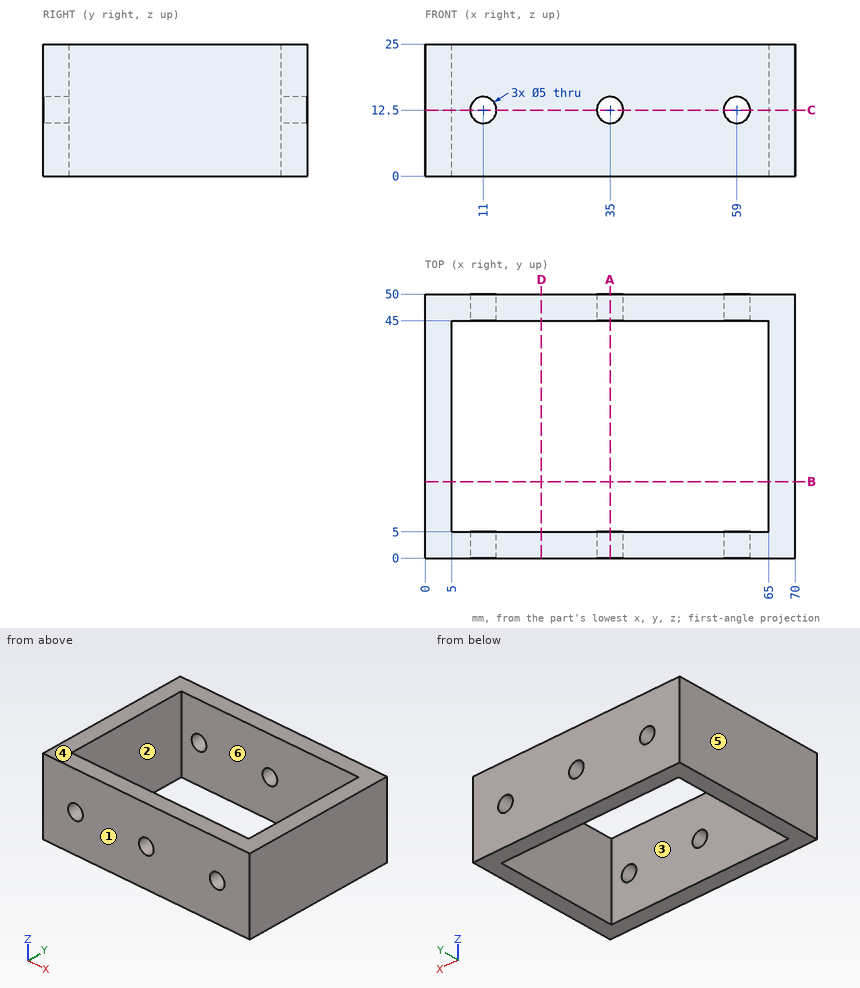
Design review of the part shown in the three views and the two pictorial views. Dimensions are in mm from the part's minimum x, y and z. A direction names the side the tool comes from. Give positions to 0.01 mm unless a question says otherwise; leave off trailing zeros. Loops run counter-clockwise (first coordinate to the right, second up) from the corner with the lowest first, then second, coordinate; pieces in that order, holes last. Notation, with made-up numbers: M 84.5,-24 L 111.5,-24 A20 ccw 111.5,-11 Z; hole C 84,22.5 d3. An arc over 180 degrees is marked long. Answer as a JSON object with one key per item and string values.
Item 1: We need section D-D (x = 22). State the section outline as (y, z) points.
Output values:
{"outline": "M 0,0 L 5,0 L 5,25 L 0,25 Z; M 45,0 L 50,0 L 50,25 L 45,25 Z"}
Item 2: We need section C-C (z = 12.5). Count the separate pieces of the cut face and the enclosed holes in it, and give its area (3 significant figures).
Output values:
{"separate pieces": "6", "enclosed holes": "0", "area": "950 mm2"}
Item 3: We need section A-A (x = 35). State the section outline as (y, z) points.
Output values:
{"outline": "M 0,0 L 5,0 L 5,10 L 0,10 Z; M 0,15 L 5,15 L 5,25 L 0,25 Z; M 45,0 L 50,0 L 50,10 L 45,10 Z; M 45,15 L 50,15 L 50,25 L 45,25 Z"}
Item 4: For P1, Ø4, axis at x = 13, z = 18, coming from the -Y side; P2, Ø4.5, axis at x = 59, z = 12.5, coming from the +Y side, all flat-tipped, find the tip position at first contact; note any pin that passes through.
Output values:
{"P1": "stops at y = 0", "P2": "passes through"}
Item 5: Mouldability with a two-part tool opening along Y and no side actions: class the marked faces 1, 2, 3 and 4 as pulls with the +Y half, pulls with the -Y half, needs draft (parallel to the pull), parting line crosses it, or undercut.
Output values:
{"face 1": "pulls with the -Y half", "face 2": "undercut", "face 3": "undercut", "face 4": "needs draft"}
Item 6: Machinability: for the marked faces 5 and 6, which of the approach directions +Z, -Z, +X, -X, +Y, -Y give a long, thin tool a straight path to every point of the face, cutting with its end or side? Answer none if there is none.
Output values:
{"face 5": "+Z, -Z, -X, +Y, -Y", "face 6": "+Z, -Z"}
Item 7: Wall thickness on line 1 along Y through (x, z) = (29.5, 12); line 2 along Z through (x, y) = (35, 46.1); line 3 along X through (y, z) = (11, 9): over which ranges is each line inside the solid? List them lowest first.
Output values:
{"line 1": "y = 0 to 5, 45 to 50", "line 2": "z = 0 to 10, 15 to 25", "line 3": "x = 0 to 5, 65 to 70"}
Item 8: We need section B-B (y = 14.5). State the section outline as (x, z) points, and give its area (3 significant figures).
Output values:
{"outline": "M 0,0 L 5,0 L 5,25 L 0,25 Z; M 65,0 L 70,0 L 70,25 L 65,25 Z", "area": "250 mm2"}
